Could you check a few things on this drawing? It's one solid part, dimensions in mm from its lowest x, y, z. Coordinates: 2 decimals unless noted, no trailing zeros. Write each loop counter-clockwise with the first axis right and the second up, starting at its lowest first coordinate (ties: lowest second). Pieces come first, ordered by that corner, then holes. Notation, with made-up numbers: M 56,44 L 113,44 A16 ccw 113,49 Z; hole C -4.5,-38 d1. An arc over 180 degrees is marked long. Use a Markdown table: item, result.
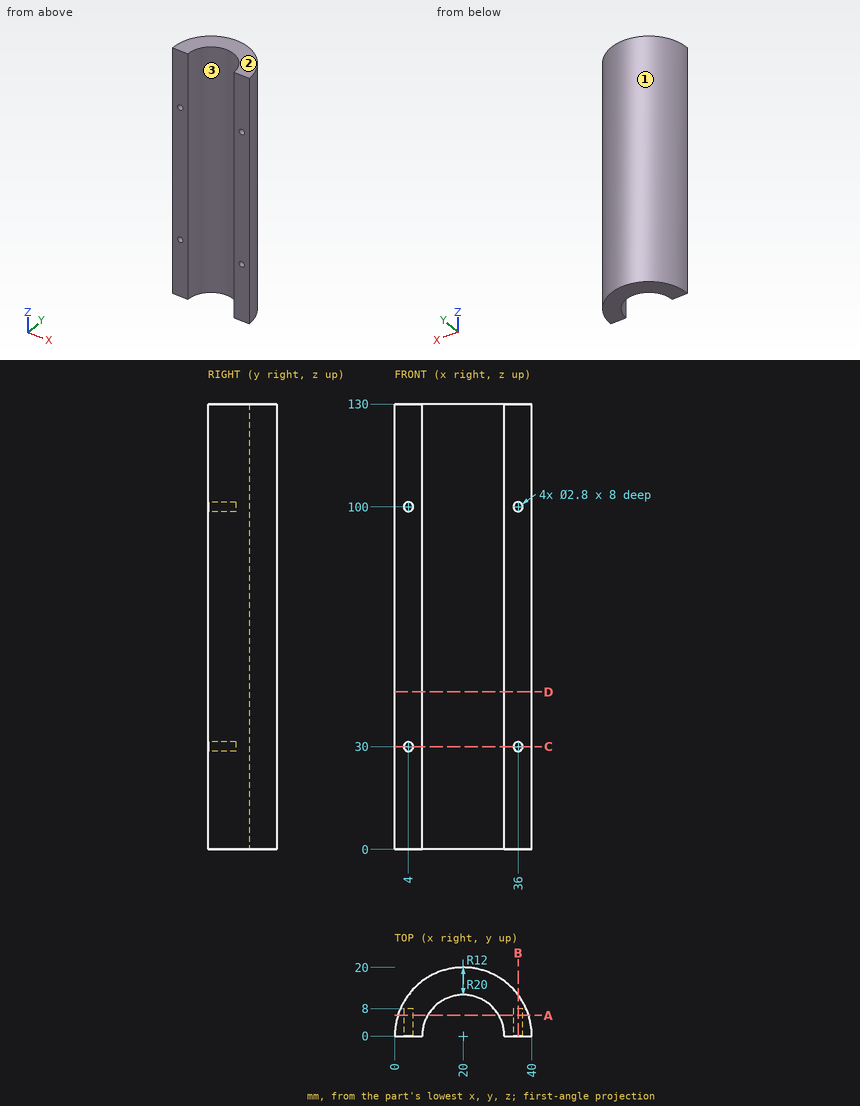
1. Suppose I cut it at D-D on z = 46. Write out the boundary of the cut face in (x, y).
Answers follow:
| item | result |
|---|---|
| outline | M 0,0 L 8,0 A12 cw 32,0 L 40,0 A20 ccw Z |
2. Suppose I cut it at B-B on x = 36. Write out the boundary of the cut face in (y, z).
Answers follow:
| item | result |
|---|---|
| outline | M 0,0 L 12,0 L 12,130 L 0,130 L 0,101.4 L 8,101.4 L 8,98.6 L 0,98.6 L 0,31.4 L 8,31.4 L 8,28.6 L 0,28.6 Z |
3. We'd pull the mould along X, two halves only. Please class the marked faces 1, 2 and 3: +X half, -X half, draft (parallel to the pull), parting line (faces both ways), or undercut.
Answers follow:
| item | result |
|---|---|
| face 1 | parting line |
| face 2 | draft |
| face 3 | undercut |
4. Will these pins go through, and if not, where does the flat tip stop? pin 1 Ø1 at (y, z) = (17.5, 75.5) entering from +X; pin 2 Ø1.5 at (y, z) = (13.5, 70.5) entering from -X; pin 3 Ø1.7 at (x, z) = (4, 30) entering from -Y.
Answers follow:
| item | result |
|---|---|
| pin 1 | stops at x = 30.54 |
| pin 2 | stops at x = 4.59 |
| pin 3 | stops at y = 8 |
5. Suppose I cut it at A-A on y = 6. Write out the boundary of the cut face in (x, z), and give its area (3 significant figures).
Answers follow:
| item | result |
|---|---|
| outline | M 0.92,0 L 9.61,0 L 9.61,130 L 0.92,130 Z; M 30.39,0 L 39.08,0 L 39.08,130 L 30.39,130 Z; hole C 4,30 d2.8; hole C 4,100 d2.8; hole C 36,30 d2.8; hole C 36,100 d2.8 |
| area | 2,230 mm2 |
6. I need wall thicknesses on probe 1 along Z at (x, y) = (4, 3); probe 2 along X at (y, z) = (1.75, 25); probe 3 along X at (y, z) = (4.25, 124.5). Which ranges of each line are inside material? Lowest first, please.
Answers follow:
| item | result |
|---|---|
| probe 1 | z = 0 to 28.6, 31.4 to 98.6, 101.4 to 130 |
| probe 2 | x = 0.08 to 8.13, 31.87 to 39.92 |
| probe 3 | x = 0.46 to 8.78, 31.22 to 39.54 |
7. Suppose I cut it at C-C on z = 30. Write out the boundary of the cut face in (x, y), and give its area (3 significant figures).
Answers follow:
| item | result |
|---|---|
| outline | M 0,0 L 2.6,0 L 2.6,8 L 5.4,8 L 5.4,0 L 8,0 A12 cw 32,0 L 34.6,0 L 34.6,8 L 37.4,8 L 37.4,0 L 40,0 A20 ccw Z |
| area | 357 mm2 |
